Could you check a few things on this model? Use its own coordinates, in mm. Face numbers are marked on the shaded views. A direction names the side the tool comes from. Round coordinates to 2 decimals unless told otherwise and drop trailing zeros. Order: outer loops, then holes, each group sorted by start corner. A loop starts at its lowest first (then second) coordinate and runs counter-clockwise, first axis right, second up. Notation, with made-up numbers: (-21.5, 4.5) -> (-3.5, 4.5) arc R24 ccw to (-3.5, 14.5) -> close; hole circle Ø5 at (61.25, 80). An arc over 180 degrees is marked (long way). Put each result on its own line as item: value. Start each with the question number.
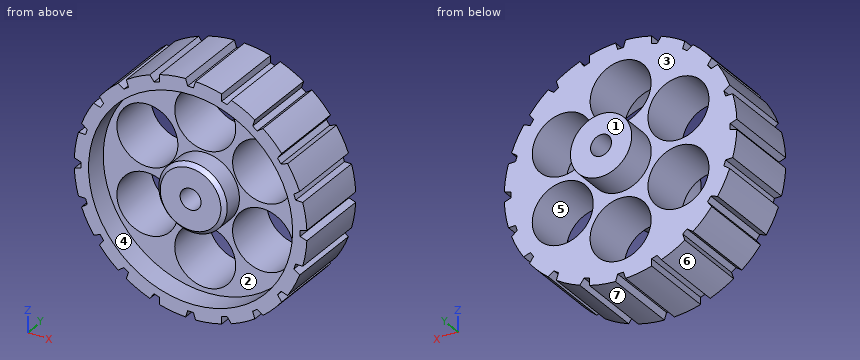
from build123d import *

# Parameters (mm, degrees)
F0_R            = 15
F0_R_2          = 1.35
F1_DEPTH        = 10
F3_R            = 3.9311890732
F4_DEPTH        = 25
F4_COPIES_COUNT = 6
F2_R            = 13.1491583338
F2_R_2          = 4.4111200255
F5_DEPTH        = 3
F6_SIZE         = 0.5
F8_DEPTH        = 10
F9_COUNT        = 20
F10_R           = 3.9505307448
F10_R_2         = 1.35
F11_DEPTH       = 4


# Not quite as in the source:
# - a pattern or mirror of a feature is missing from the dataset's text; its kind, count and spacing are read off the source's solid
# - a feature names something its author has since deleted; it is built from what else it names


with BuildPart() as f1:
    # F0 (on Front) → F1 (new body)
    with BuildSketch(Plane.XZ):
        Circle(F0_R)
        Circle(F0_R_2, mode=Mode.SUBTRACT)
    extrude(amount=F1_DEPTH)

    # F3 (on face) → F4 (cut)
    with BuildSketch(Plane.XZ.offset(10)):
        with Locations((0, 8.6101097986)):
            Circle(F3_R)
    f4 = extrude(amount=-F4_DEPTH, mode=Mode.SUBTRACT)

    # F4_copies: F4 ×6 about axis
    f4_copies_axis = Axis((0, 0, 0), (0, 1, 0))
    for i in range(1, F4_COPIES_COUNT):
        add(f4.rotate(f4_copies_axis, i * 360 / F4_COPIES_COUNT), mode=Mode.SUBTRACT)

    # F2 (on face) → F5 (cut)
    with BuildSketch(Plane.XZ.offset(10)):
        Circle(F2_R)
        Circle(F2_R_2, mode=Mode.SUBTRACT)
    extrude(amount=-F5_DEPTH, mode=Mode.SUBTRACT)

    # F6
    f6_edges = [f1.edges().sort_by_distance(p)[0] for p in [
        (-4.41112, -10, 0),
    ]]
    chamfer(f6_edges, length=F6_SIZE)

    # F7 (on face) → F8 (cut)
    with BuildSketch(Plane.XZ.offset(10)):
        with BuildLine():
            ThreePointArc((0.6504242485, 14.9858916417), (0, 15), (-0.6504242485, 14.9858916417))
            Line((-0.6504242485, 14.9858916417), (-0.3680477384, 14.1178695485))
            Line((-0.3680477384, 14.1178695485), (0, 14.1178695485))
            Line((0, 14.1178695485), (0.3680477384, 14.1178695485))
            Line((0.3680477384, 14.1178695485), (0.6504242485, 14.9858916417))
        make_face()
    f8 = extrude(amount=-F8_DEPTH, mode=Mode.SUBTRACT)

    # F9: F8 ×20 about axis
    f9_axis = Axis((0, 0, 0), (0, 1, 0))
    for i in range(1, F9_COUNT):
        add(f8.rotate(f9_axis, i * 360 / F9_COUNT), mode=Mode.SUBTRACT)

    # F10 (on face) → F11 (join)
    with BuildSketch(Plane(origin=(0, 0, 0), x_dir=(-1, 0, 0), z_dir=(0, 1, 0))):
        Circle(F10_R)
        Circle(F10_R_2, mode=Mode.SUBTRACT)
    extrude(amount=F11_DEPTH)


solid = f1.part
1. I need wall thicknesses on L1, parallel to Z at x = 0, y = -5.25; L2, parallel to Z at x = -8.5, y = -3.25; L3, parallel to X at y = -2.75, z = 6.5. Which ranges of each line are inside material? Lowest first, please.
2. If we section it at D-D, the plane z = -6: Please give me the cut outline in (x, y).
3. If we section it at A-A, the plane x = 0: Count the separate pieces of the cut face and the enclosed holes in it, then the cut area to 3 significant figures.
4. Which directions (+Z, -Z, +X, -X, +Y, -Y) give clear straight access to the entire face, cutting with the end or side of a thin tool? Please do the marked faces 1, 2 and 3.
5. Thinking about a two-plate mould opening in X: for the marked faces 4, 5, 6 and 7, which applies, +X half, -X half, draft (parallel to the pull), parting line (faces both ways), or undercut?
6. If we section it at B-B, the plane z = 0: Please give me the cut outline in (x, y), then the cut area to 3 significant figures.
7. For pin 1 Ø8 at (x, y) = (-7.5, 0) entering from -Z; pin 2 Ø6.5 at (x, z) = (0, 8.61) entering from -Y; pin 3 Ø3 at (y, z) = (1, -3.5) entering from -X; pin 4 Ø0.6 at (x, y) = (0, -4) entering from -Z, each with a flat end and sliding along its axis, tell me the tip position at first contact or that it passes through.
Results below:
1. L1: -14.12 to -12.54, -4.68 to -1.35, 1.35 to 4.68, 12.54 to 14.12
1. L2: -11.28 to -8.1, -0.51 to 0.51, 8.1 to 11.28
1. L3: -13.52 to -10.72, -4.2 to -3.32, 3.32 to 4.2, 10.72 to 13.52
2. outline: (-13.75, -10) -> (-11.7, -10) -> (-11.7, -7) -> (-11, -7) -> (-11, 0) -> (-13.75, 0) -> close; (-3.91, -7) -> (-2.94, -7) -> (-2.94, 0) -> (-3.91, 0) -> close; (2.94, -7) -> (3.91, -7) -> (3.91, 0) -> (2.94, 0) -> close; (11, -7) -> (11.7, -7) -> (11.7, -10) -> (13.75, -10) -> (13.75, 0) -> (11, 0) -> close
3. separate pieces: 4
3. enclosed holes: 0
3. area: 113 mm2
4. face 1: +Z, -Z, +X, -X, +Y
4. face 2: -Y
4. face 3: +Y
5. face 4: undercut
5. face 5: undercut
5. face 6: -X half
5. face 7: +X half
6. outline: (-14.12, -10) -> (-13.15, -10) -> (-13.15, -7) -> (-4.41, -7) -> (-4.41, -9.5) -> (-3.91, -10) -> (-1.35, -10) -> (-1.35, 4) -> (-3.95, 4) -> (-3.95, 0) -> (-14.12, 0) -> close; (1.35, -10) -> (3.91, -10) -> (4.41, -9.5) -> (4.41, -7) -> (13.15, -7) -> (13.15, -10) -> (14.12, -10) -> (14.12, 0) -> (3.95, 0) -> (3.95, 4) -> (1.35, 4) -> close
6. area: 223 mm2
7. pin 1: z = -14.59
7. pin 2: through
7. pin 3: x = -14.81
7. pin 4: z = -14.12
